Design review of the part built by this model. Coordinates are the model's own, in mm. Round coordinates to 2 decimals unless told otherwise and drop trailing zeros. Loops run counter-clockwise (first coordinate to the right, second up) from the corner with the lowest first, then second, coordinate; pieces in that order, holes last. Notation, with made-up numbers: M 53,-20 L 79,-20 A26 ccw 79,2 Z; hole C 14.5,39 d10. An arc over 180 degrees is marked long. Use a Markdown table: item, result.
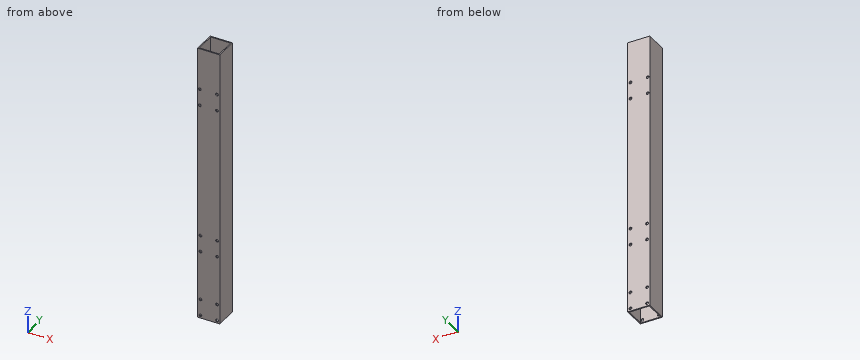
from build123d import *

# Parameters (mm, degrees)
F0_W     = 100
F0_H     = 100
F0_W_2   = 90
F0_H_2   = 90
F1_DEPTH = 1265
F3_D     = 12.5
F5_D     = 12.5


with BuildPart() as f1:
    # F0 (on Top) → F1 (new body)
    with BuildSketch(Plane.XY):
        Rectangle(F0_W, F0_H)
        Rectangle(F0_W_2, F0_H_2, mode=Mode.SUBTRACT)
    extrude(amount=F1_DEPTH)

    # F3 (through all)
    with Locations(Plane.XZ.offset(50)):
        with Locations((-37.5, 387.5), (37.5, 387.5), (37.5, 312.5), (-37.5, 312.5), (-37.5, 87.5), (-37.5, 12.5), (37.5, 87.5), (37.5, 12.5)):
            Hole(F3_D / 2)

    # F5 (through all)
    with Locations(Plane.XZ.offset(50)):
        with Locations((-40.149868, 999.03965), (37.251893, 999.03965), (-40.149868, 1074.598551), (37.251893, 1074.598551)):
            Hole(F5_D / 2)


solid = f1.part
1. Take a section at A-A on x = 5. Give the boundary of the cut face in (y, z), and give its area (4 significant figures).
Check values:
| item | result |
|---|---|
| outline | M -50,0 L -45,0 L -45,1265 L -50,1265 Z; M 45,0 L 50,0 L 50,1265 L 45,1265 Z |
| area | 12,650 mm² |
2. Wall thickness on line 1 along X through (y, z) = (-48.75, 387.5); line 2 along Y through (x, z) = (-29, 1184.5): over which ranges is each line inside the solid? List them lowest first. Write a range as from..to.
Check values:
| item | result |
|---|---|
| line 1 | x = -50..-43.75, -31.25..31.25, 43.75..50 |
| line 2 | y = -50..-45, 45..50 |
3. Take a section at B-B on y = -9. Give the boundary of the cut face in (x, z), and give its area (3 significant figures).
Check values:
| item | result |
|---|---|
| outline | M -50,0 L -45,0 L -45,995.1 A6.25 cw -45,1002.98 L -45,1070.66 A6.25 cw -45,1078.54 L -45,1265 L -50,1265 Z; M 45,0 L 50,0 L 50,1265 L 45,1265 Z |
| area | 12,600 mm² |
